Verification items for the finished model (mm, model axes). Face numbers are marked on the shaded views. Coordinates: 2 decimals unless noted, no trailing zeros. Answer as a JSON object with one key per item and string values. Group by question number.
Q1. Gauge pin test, flat ends, axial feed: pin 1 Ø3 at (y, z) = (2.5, 20) entering from -X; pin 2 Ø2 at (y, z) = (0.5, -12) entering from +X; pin 3 Ø8 at (x, z) = (25.5, 25) entering from -Y; pin 4 Ø16 at (x, z) = (-1, 0.5) entering from +Y. Record the tip position at first contact, or that the pin passes through.
Q2. Release check for a two-part mould opening along Z. For the marked faces 1 and 2 record: released by +Z, released by -Z, zero draft, split by the parting line, or undercut.
Q3. Cross-section at A-A on z = 0. Give the number of separate pieces and of enclosed holes in the cut face, and give its area (4 significant figures).
Q4. Scan lines: L1, parallel to Z at x = 9, y = 2.25; L2, parallel to Z at x = 2, y = 3; L3, parallel to X at y = 1, z = 4. Record each from-to range of solid material in increasing order.
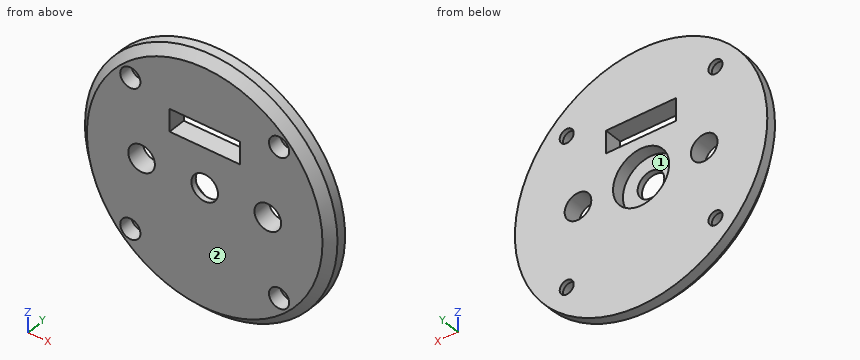
Autodesk Inventor part; units mm, degrees
ref_plane "YZ Plane" through (0, 0, 0) normal (1, 0, 0) x (0, 1, 0)
ref_plane "XZ Plane" through (0, 0, 0) normal (0, 1, 0) x (-1, 0, 0)
ref_plane "XY Plane" through (0, 0, 0) normal (0, 0, 1) x (1, 0, 0)
sketch "Sketch1" plane through (0, 0, 0) normal (0, 1, 0) x (-1, 0, 0)
  circle A0 centre (0, 0) radius 45
  circle A1 centre (0, 0) radius 10
  circle A2 centre (22.5, 0) radius 4.75
  circle A3 centre (-22.5, 0) radius 4.75
  line L0 (0, -25.6154) -> (0, 19.3488) construction
  circle A4 centre (0, 0) radius 4.75
  line L1 (12.5, 22) -> (-12.5, 22)
  line L2 (-12.5, 22) -> (-12.5, 14)
  line L3 (-12.5, 14) -> (12.5, 14)
  line L4 (12.5, 14) -> (12.5, 22)
  line L5 (12.5, 22) -> (-12.5, 14) construction
  line L6 (-12.5, 22) -> (12.5, 14) construction
  point P0 (0, 18)
  dimension "d0" = 90
  dimension "d1" = 20
  dimension "d2" = 45
  dimension "d20" = 18
  dimension "d21" = 8
  dimension "d22" = 25
  dimension "d26" = 9.5
extrude "Extrusion1" add sketch "Sketch1" against normal blind 2 contours A0 | A1
extrude "Extrusion2" add sketch "Sketch1" along normal blind 4.5 contours A0
sketch "Sketch2" plane through (0, -2, 0) normal (0, -1, 0) x (1, 0, 0)
  line L0 (26.5165, -26.5165) -> (0, 0) construction
  line L1 (17.2429, 0) -> (-14.3285, 0) construction
  line L2 (0, -10.0849) -> (0, 10.0849) construction
  point P0 (-26.5165, -26.5165)
  point P1 (26.5165, 26.5165)
  point P2 (-26.5165, 26.5165)
  dimension "d9" = 37.5
  dimension "d10" = 45
hole "Hole1" at (26.5165, -2, -26.5165) at (-26.5165, -2, -26.5165) at (26.5165, -2, 26.5165) at (-26.5165, -2, 26.5165) direction (0, 1, 0) diameter 5 end through all counterbore diameter 7.2 counterbore depth 5
chamfer "Chamfer1" distance 3 angle 45 1 edges at (45, -2, 0)
properties part number "SCARA swivel top - lid"
Computed values:
{
 "1": {"pin 1": "stops at x = -41.02", "pin 2": "stops at x = 43.6", "pin 3": "stops at y = -2", "pin 4": "stops at y = 0"},
 "2": {"face 1": "undercut", "face 2": "zero draft"},
 "3": {"separate pieces": "4", "enclosed holes": "0", "area": "343.5 mm²"},
 "4": {"L1": "z = -44.09 to -4.36, 4.36 to 14, 22 to 44.09", "L2": "z = -44.96 to -9.8, 9.8 to 14, 22 to 44.96", "L3": "x = -44.82 to -25.06, -19.94 to -9.17, 9.17 to 19.94, 25.06 to 44.82"}
}
